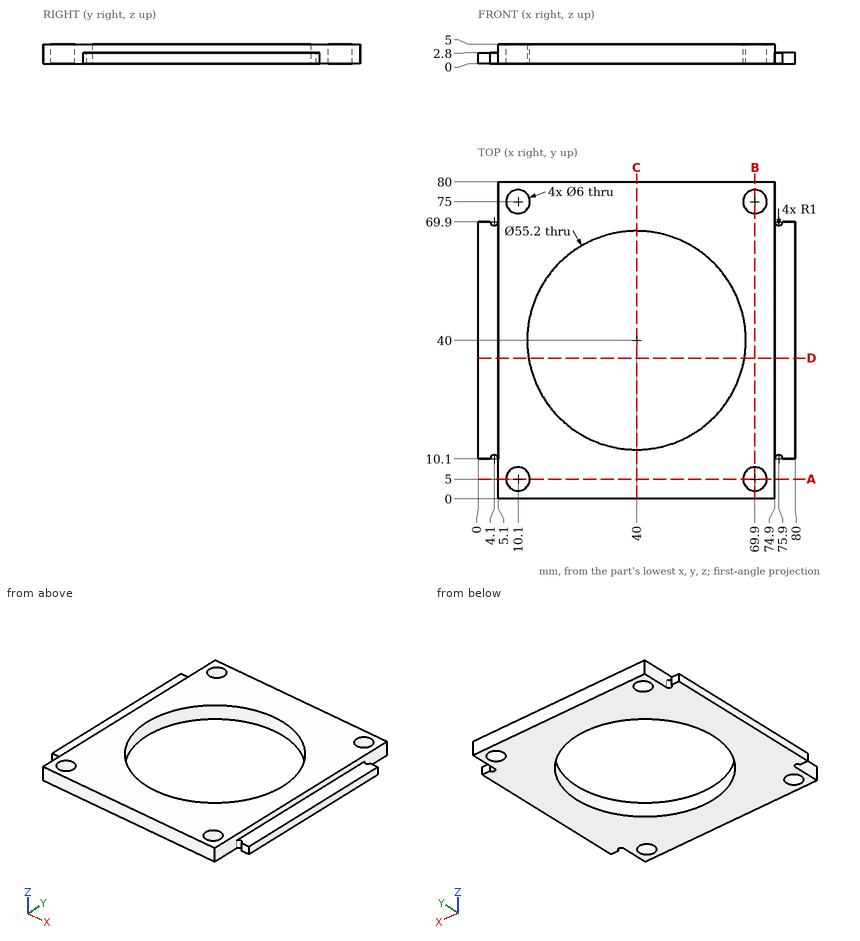
Here's the drawing with two shaded views (mm, measured from the low corner). I have some questions. Coordinates: 2 decimals unless noted, no trailing zeros. Loops run counter-clockwise (first coordinate to the right, second up) from the corner with the lowest first, then second, coordinate; pieces in that order, holes last.
Item 1: Suppose I cut it at B-B (x = 69.9). Please give me the cut outline in (y, z), then the cut area to 3 significant figures.
Answers below:
outline: (0, 0) - (2, 0) - (2, 5) - (0, 5) - close; (8, 0) - (72, 0) - (72, 5) - (8, 5) - close; (78, 0) - (80, 0) - (80, 5) - (78, 5) - close
area: 340 mm2
Item 2: Please list where these lines run through material, in increasing order: L1, parallel to X at y = 5, z = 1.4; L2, parallel to Y at x = 69.9, z = 2.3; L3, parallel to Y at x = 41, z = 2.4.
Answers below:
L1: x = 5.1 to 7.1, 13.1 to 66.9, 72.9 to 74.9
L2: y = 0 to 2, 8 to 72, 78 to 80
L3: y = 0 to 12.42, 67.58 to 80
Item 3: I'm going to push flat-ended pins straight in: pin 1 (3 mm diameter, centred on x = 78.5, z = 1, fed in from +Y); pin 2 (4 mm diameter, centred on x = 2, y = 53, fed in from +Z); pin 3 (2 mm diameter, centred on x = 2, z = 1, fed in from -Y). Where does each tip first touch, or does it pass through?
Answers below:
pin 1: stops at y = 69.9
pin 2: stops at z = 2.8
pin 3: stops at y = 10.1
Item 4: Suppose I cut it at C-C (x = 40). Please give me the cut outline in (y, z).
Answers below:
outline: (0, 0) - (12.4, 0) - (12.4, 5) - (0, 5) - close; (67.6, 0) - (80, 0) - (80, 5) - (67.6, 5) - close
Item 5: Suppose I cut it at A-A (y = 5). Please give me the cut outline in (x, z), then the cut area to 3 significant figures.
Answers below:
outline: (5.1, 0) - (7.1, 0) - (7.1, 5) - (5.1, 5) - close; (13.1, 0) - (66.9, 0) - (66.9, 5) - (13.1, 5) - close; (72.9, 0) - (74.9, 0) - (74.9, 5) - (72.9, 5) - close
area: 289 mm2
Item 6: Suppose I cut it at D-D (y = 35.5). Please give me the cut outline in (x, z), then the cut area to 3 significant figures.
Answers below:
outline: (0, 0) - (12.77, 0) - (12.77, 5) - (5.1, 5) - (5.1, 2.8) - (0, 2.8) - close; (67.23, 0) - (80, 0) - (80, 2.8) - (74.9, 2.8) - (74.9, 5) - (67.23, 5) - close
area: 105 mm2
